Autodesk Inventor part; units mm, degrees
ref_plane "YZ Plane" through (0, 0, 0) normal (1, 0, 0) x (0, 1, 0)
ref_plane "XZ Plane" through (0, 0, 0) normal (0, 1, 0) x (-1, 0, 0)
ref_plane "XY Plane" through (0, 0, 0) normal (0, 0, 1) x (1, 0, 0)
sketch "Skizze1" plane through (0, 0, 0) normal (0, 1, 0) x (-1, 0, 0)
  arc A0 (349.7617, -93.7184) -> (349.7617, 93.7184) centre (0, 0) ccw
  arc A1 (357.296, -95.7372) -> (357.296, 95.7372) centre (0, 0) ccw
  line L0 (357.296, 95.7372) -> (0, 0) construction
  line L1 (0, 0) -> (357.296, -95.7372) construction
  line L2 (444.782, 0) -> (-74.1303, 0) construction
  line L3 (357.296, 95.7372) -> (349.7617, 93.7184)
  line L4 (357.296, -95.7372) -> (349.7617, -93.7184)
  line L5 (361.1319, 80.061) -> (0, 0) construction
  line L6 (369.5479, 16.1348) -> (0, 0) construction
  line L7 (369.5479, -16.1348) -> (0, 0) construction
  line L8 (361.1319, -80.061) -> (0, 0) construction
  arc A2 (353.5289, -94.7278) -> (353.5289, 94.7278) centre (0, 0) ccw construction
  circle A3 centre (357.3243, 79.2169) radius 1.6
  circle A4 centre (365.6516, 15.9647) radius 1.6
  circle A5 centre (365.6516, -15.9647) radius 1.6
  circle A6 centre (357.3243, -79.2169) radius 1.6
  circle A7 centre (357.3243, 79.2169) radius 3
  circle A8 centre (365.6516, 15.9647) radius 3
  circle A9 centre (365.6516, -15.9647) radius 3
  circle A10 centre (357.3243, -79.2169) radius 3
  arc A11 (360.4527, 83.0652) -> (352.8301, 81.4083) centre (358.5974, 73.2389) ccw
  arc A12 (354.1773, 75.3315) -> (361.786, 77.0512) centre (355.9517, 85.1728) ccw
  arc A13 (369.4008, 19.2113) -> (361.6062, 18.9032) centre (365.8673, 9.8564) ccw
  arc A14 (361.8777, 12.6848) -> (369.6695, 13.0572) centre (365.3341, 22.0685) ccw
  arc A15 (369.6695, -13.0572) -> (361.8777, -12.6848) centre (365.3341, -22.0685) ccw
  arc A16 (361.786, -77.0512) -> (354.1773, -75.3315) centre (355.9517, -85.1728) ccw
  arc A17 (352.8301, -81.4083) -> (360.4527, -83.0652) centre (358.5974, -73.2389) ccw
  arc A18 (361.6062, -18.9032) -> (369.4008, -19.2113) centre (365.8673, -9.8564) ccw
  circle A19 centre (357.3243, -79.2169) radius 5 construction
  circle A20 centre (365.6516, -15.9647) radius 5 construction
  circle A21 centre (365.6516, 15.9647) radius 5 construction
  circle A22 centre (357.3243, 79.2169) radius 5 construction
  dimension "d1" = 7.8
  dimension "d18" = 366
  dimension "d19" = 10
  dimension "d2" = 30
  dimension "d4" = 10
  dimension "d5" = 5
  dimension "d6" = 10
  dimension "d7" = 3.2
  dimension "d8" = 6
  dimension "d17" = 10
extrude "Extrusion1" add sketch "Skizze1" against normal blind 6 contours A0 A17 A1 L4 | A0 A16 A1 A17 | A0 A18 A1 A16 | A0 A15 A1 A18 | A0 A14 A1 A15 | A0 A13 A1 A14 | A0 A12 A1 A13 | A0 A11 A1 A12 | A0 L3 A1 A11 | A7 | A8 | A9 | A10
extrude "Extrusion2" add sketch "Skizze1" along normal blind 3 contours A0 A17 A1 L4 | A0 A18 A1 A16 | A0 A14 A1 A15 | A0 A12 A1 A13 | A0 L3 A1 A11
chamfer "Fase1" distance 1 angle 45 8 edges at (-362.1, -6, 0) (-349.7617, -1.5, 93.7184) (-357.296, -1.5, 95.7372) (-349.7617, -1.5, -93.7184) (-357.296, -1.5, -95.7372) (-369.9, -6, 0) (-353.5289, -6, -94.7278) (-353.5289, -6, 94.7278)
properties part number "LED-Ring_Connector_v2"
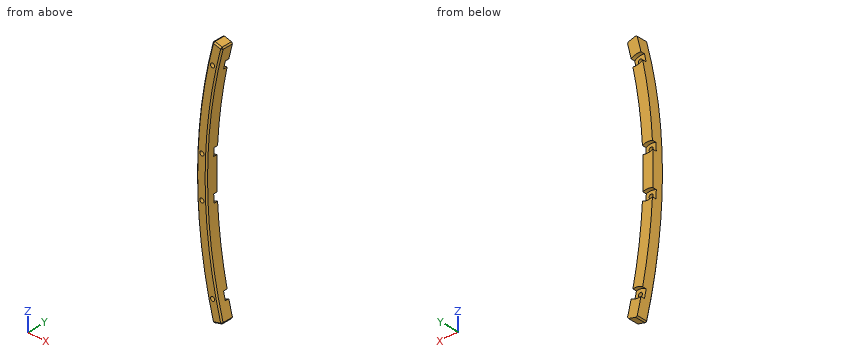
Source: CAD feature listing. Evaluate the final solid. Frame: model axes, mm. Round coordinates to 2 decimals unless told otherwise and drop trailing zeros. Loops run counter-clockwise (first coordinate to the right, second up) from the corner with the lowest first, then second, coordinate; pieces in that order, holes last.
Q1. Section A-A, the plane y = 1.5. Return loops of the section in (x, z), plus the area to 3 significant figures.
Q2. Ray query, line 1 (Z direction, x = -353.75, y = 2.5); line 2 (X direction, y = 0.5, z = -3.5); line 3 (X direction, y = 0.75, z = 37.5). Return the intervals inside material, ascending.
Q3. First-contact query: P1, Ø6, axis at x = -364.5, z = -16.5, coming from the +Y side; P2, Ø4, axis at y = 2, z = 63, coming from the -X side. Flat tips, straight axial feed; report the tip coordinate or a pass-through.
Solutions:
1. outline: (-369.67, -13.06) arc R10 cw to (-361.88, -12.68) arc R362.1 cw to (-361.88, 12.68) arc R10 cw to (-369.67, 13.06) arc R369.9 ccw to start; (-369.4, -19.21) arc R369.9 ccw to (-361.79, -77.05) arc R10 cw to (-354.18, -75.33) arc R362.1 cw to (-361.61, -18.9) arc R10 cw to start; (-369.4, 19.21) arc R10 cw to (-361.61, 18.9) arc R362.1 cw to (-354.18, 75.33) arc R10 cw to (-361.79, 77.05) arc R369.9 ccw to start; (-360.45, -83.07) arc R369.9 ccw to (-357.55, -94.77) - (-356.33, -95.48) - (-350.73, -93.98) - (-350.02, -92.75) arc R362.1 cw to (-352.83, -81.41) arc R10 cw to start; (-360.45, 83.07) arc R10 cw to (-352.83, 81.41) arc R362.1 cw to (-350.02, 92.75) - (-350.73, 93.98) - (-356.33, 95.48) - (-357.55, 94.77) arc R369.9 ccw to start
1. area: 1,270 mm2
2. line 1: z = -94.79 to -81.99, 81.99 to 94.79
2. line 2: x = -369.88 to -362.08
2. line 3: x = -367.99 to -360.15
3. P1: stops at y = 0
3. P2: stops at x = -364.84
